Source: CAD feature listing. Evaluate the final solid. Frame: model axes, mm. Face numbers are marked on the shaded views. Coordinates: 2 decimals unless noted, no trailing zeros. Loops run counter-clockwise (first coordinate to the right, second up) from the corner with the lowest first, then second, coordinate; pieces in that order, holes last.
Item 1: Section query B-B, the plane z = 30. Return the cut outline in (x, y), then the cut area to 3 significant figures.
Item 2: Line query: probe 1 along X at (y, z) = (26.4, 10); probe 2 along Z at (x, y) = (-0.5, 30.25); probe 3 along X at (y, z) = (31, 46.5). Output: solid intervals per line, ascending.
Item 3: Pin query (flat end, axial travel): pin 1 Ø7.5 at (x, z) = (0, 50) entering from -Y; pin 2 Ø4 at (y, z) = (29.5, 15) entering from +X; pin 3 Ø7.5 at (x, z) = (0, 10) entering from +Y; pin 4 Ø1 at (y, z) = (27, 8.5) entering from -X. Return the tip coordinate at first contact, or that it passes through.
Item 4: Section query C-C, the plane y = 29. State how many separate pieces and enclosed holes the cut face has, then the cut area to 3 significant figures.
Item 5: Section query A-A, the plane x = 0. Return the cut outline in (y, z).
Item 6: Pull-direction query (X, two-part tool) for the marked faces 1, 2 and 3; classes: +X half, -X half, draft (parallel to the pull), parting line (faces both ways), or undercut.
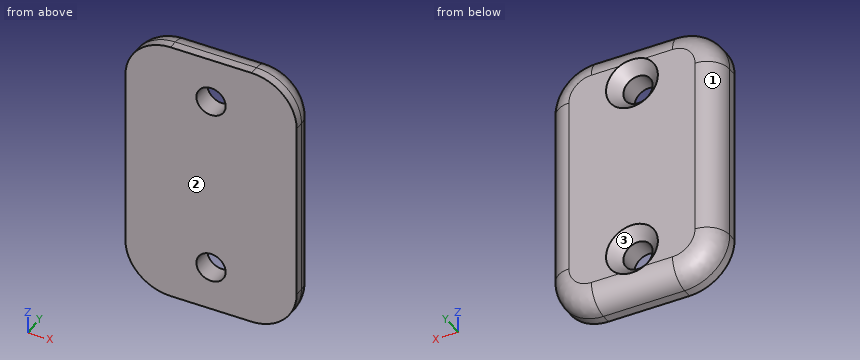
```python
from build123d import *

# Parameters (mm, degrees)
SKETCH1_W           = 43
SKETCH1_H           = 43
SKETCH1_R           = 13.75
SKETCH1_H_2         = 7
BOSS_EXTRUDE1_DEPTH = 60
SKETCH3_R           = 3.25
CUT_EXTRUDE5_DEPTH  = 85.038324591
CHAMFER2_SIZE       = 2.5
CUT_EXTRUDE6_START  = -38
CUT_EXTRUDE6_DEPTH  = 15
SKETCH9_W           = 10
SKETCH9_H           = 51.2
CUT_EXTRUDE7_DEPTH  = 75.012431469
FILLET1_R           = 5
FILLET2_R           = 10


with BuildPart() as part:
    # Sketch1 → Boss-Extrude1 (new body)
    # profile 1 of 3: a face of its own
    with BuildSketch(Plane.XY):
        with Locations((2.5, 2.5)):
            Rectangle(SKETCH1_W, SKETCH1_H)
        Circle(SKETCH1_R, mode=Mode.SUBTRACT)
    # profile 2 of 3: a face of its own
    with BuildSketch(Plane.XY):
        with Locations((2.5, 28.7)):
            Rectangle(SKETCH1_W, SKETCH1_H_2)
    # profile 3 of 3: a face of its own
    with BuildSketch(Plane.XY):
        Polygon((24, 24), (24, -19), (29, -19), (29, 32.2), (24, 32.2), (24, 25.2), align=None)
    extrude(amount=BOSS_EXTRUDE1_DEPTH)

    # Sketch3 → Cut-Extrude5 (cut, through all)
    with BuildSketch(Plane(origin=(0, 32.2, 0), x_dir=(1, 0, 0), z_dir=(0, 1, 0))):
        with Locations(Location((0, -50, 0), (0, 0, 270))):
            Circle(SKETCH3_R)
        with Locations(Location((0, -10, 0), (0, 0, 270))):
            Circle(SKETCH3_R)
    extrude(amount=-CUT_EXTRUDE5_DEPTH, mode=Mode.SUBTRACT)

    # Chamfer2
    chamfer2_edges = [part.edges().sort_by_distance(p)[0] for p in [
        (0, 32.2, 46.75),
        (0, 32.2, 6.75),
    ]]
    chamfer(chamfer2_edges, length=CHAMFER2_SIZE)

    # Sketch7 → Cut-Extrude6 (cut)
    with BuildSketch(Plane.XZ.offset(19).offset(CUT_EXTRUDE6_START)):
        Polygon((0, 43.533676985), (5.6, 46.766838493), (5.6, 53.233161507), (0, 56.466323015), (-5.6, 53.233161507), (-5.6, 46.766838493), align=None)
        Polygon((-5.6, 13.233161507), (0, 16.466323015), (5.6, 13.233161507), (5.6, 6.766838493), (0, 3.533676985), (-5.6, 6.766838493), align=None)
    extrude(amount=CUT_EXTRUDE6_DEPTH, mode=Mode.SUBTRACT)

    # Sketch9 → Cut-Extrude7 (cut, through all)
    with BuildSketch(Plane(origin=(0, 0, 0), x_dir=(-1, 0, 0), z_dir=(0, 0, -1))):
        with Locations((-24, 6.6)):
            Rectangle(SKETCH9_W, SKETCH9_H)
    extrude(amount=-CUT_EXTRUDE7_DEPTH, mode=Mode.SUBTRACT)


with BuildPart() as body_2:
    # of the pieces the cut leaves, the one that is kept (cut_extrude7_keep)
    add(part.part.solids().sort_by_distance((-19, 32.2, 0))[0])

    # Fillet1
    # the kernel refuses this fillet: 5 mm, written as the material it takes off along each edge
    with BuildSketch(Plane(origin=(-31.5, 32.2, 0), x_dir=(0, 0, 1), z_dir=(1, 0, 0)), Plane(origin=(31.5, 32.2, 60), x_dir=(0, 0, -1), z_dir=(-1, 0, 0))) as fillet1_piece_1:
        with BuildLine():
            CenterArc((FILLET1_R, FILLET1_R), FILLET1_R, 180, 90)
            Line((0, FILLET1_R), (0, 0))
            Line((0, 0), (FILLET1_R, 0))
        make_face()
    extrude(amount=63, mode=Mode.SUBTRACT)
    with BuildSketch(Plane(origin=(-19, 32.2, -12.5), x_dir=(1, 0, 0), z_dir=(0, 0, 1))) as fillet1_piece_2:
        with BuildLine():
            CenterArc((FILLET1_R, -FILLET1_R), FILLET1_R, 90, 90)
            Line((0, -FILLET1_R), (0, 0))
            Line((0, 0), (FILLET1_R, 0))
        make_face()
    extrude(amount=85, mode=Mode.SUBTRACT)
    with BuildSketch(Plane(origin=(19, 32.2, -12.5), x_dir=(-1, 0, 0), z_dir=(0, 0, 1))) as fillet1_piece_3:
        with BuildLine():
            CenterArc((FILLET1_R, FILLET1_R), FILLET1_R, 180, 90)
            Line((0, FILLET1_R), (0, 0))
            Line((0, 0), (FILLET1_R, 0))
        make_face()
    extrude(amount=85, mode=Mode.SUBTRACT)

    # Fillet2
    # the kernel refuses this fillet: 10 mm, written as the material it takes off along each edge
    with BuildSketch(Plane(origin=(-9, 32.2, 10), x_dir=(0, 0, -1), z_dir=(1, 0, 0))) as fillet2_piece_1:
        with BuildLine():
            CenterArc((5, -5), 5, 0, 90)
            Line((10, -5), (10, 0))
            Line((10, 0), (5, 0))
        make_face()
    revolve(axis=Axis((-9, 32.2, 10), (0, 1, 0)), revolution_arc=90, mode=Mode.SUBTRACT)
    with BuildSketch(Plane(origin=(9, 32.2, 10), x_dir=(1, 0, 0), z_dir=(0, 0, 1))) as fillet2_piece_2:
        with BuildLine():
            CenterArc((5, -5), 5, 0, 90)
            Line((10, -5), (10, 0))
            Line((10, 0), (5, 0))
        make_face()
    revolve(axis=Axis((9, 32.2, 10), (0, 1, 0)), revolution_arc=90, mode=Mode.SUBTRACT)
    with BuildSketch(Plane(origin=(-9, 32.2, 50), x_dir=(-1, 0, 0), z_dir=(0, 0, -1))) as fillet2_piece_3:
        with BuildLine():
            CenterArc((5, -5), 5, 0, 90)
            Line((10, -5), (10, 0))
            Line((10, 0), (5, 0))
        make_face()
    revolve(axis=Axis((-9, 32.2, 50), (0, 1, 0)), revolution_arc=90, mode=Mode.SUBTRACT)
    with BuildSketch(Plane(origin=(9, 32.2, 50), x_dir=(0, 0, 1), z_dir=(-1, 0, 0))) as fillet2_piece_4:
        with BuildLine():
            CenterArc((5, -5), 5, 0, 90)
            Line((10, -5), (10, 0))
            Line((10, 0), (5, 0))
        make_face()
    revolve(axis=Axis((9, 32.2, 50), (0, 1, 0)), revolution_arc=90, mode=Mode.SUBTRACT)
    with BuildSketch(Plane(origin=(19, 32.2, 0), x_dir=(0, 0, 1), z_dir=(0, -1, 0)), Plane(origin=(-19, 32.2, 60), x_dir=(0, 0, -1), z_dir=(0, -1, 0))) as fillet2_piece_5:
        with BuildLine():
            CenterArc((FILLET2_R, FILLET2_R), FILLET2_R, 180, 90)
            Line((0, FILLET2_R), (0, 0))
            Line((0, 0), (FILLET2_R, 0))
        make_face()
    extrude(amount=32, mode=Mode.SUBTRACT)
    with BuildSketch(Plane(origin=(19, 0.2, 60), x_dir=(-1, 0, 0), z_dir=(0, 1, 0)), Plane(origin=(-19, 32.2, 0), x_dir=(0, 0, 1), z_dir=(0, -1, 0))) as fillet2_piece_6:
        with BuildLine():
            CenterArc((FILLET2_R, -FILLET2_R), FILLET2_R, 90, 90)
            Line((0, -FILLET2_R), (0, 0))
            Line((0, 0), (FILLET2_R, 0))
        make_face()
    extrude(amount=32, mode=Mode.SUBTRACT)


solid = body_2.part
```
Verdict:
1. outline: (-19, 25.2) - (19, 25.2) - (19, 27.2) arc R5 ccw to (14, 32.2) - (-14, 32.2) arc R5 ccw to (-19, 27.2) - close
1. area: 255 mm2
2. probe 1: x = -19 to -3.25, 3.25 to 19
2. probe 2: z = 1.04 to 6.23, 13.77 to 46.23, 53.77 to 58.96
2. probe 3: x = -17.25 to -2.91, 2.91 to 17.25
3. pin 1: stops at y = 25.2
3. pin 2: stops at x = 18.99
3. pin 3: stops at y = 30.2
3. pin 4: stops at x = -18.95
4. separate pieces: 1
4. enclosed holes: 2
4. area: 2,070 mm2
5. outline: (25.2, 0) - (27.2, 0) arc R5 ccw to (32.15, 4.3) - (29.7, 6.75) - (25.2, 6.75) - close; (25.2, 13.25) - (29.7, 13.25) - (32.2, 15.75) - (32.2, 44.25) - (29.7, 46.75) - (25.2, 46.75) - close; (25.2, 53.25) - (29.7, 53.25) - (32.15, 55.7) arc R5 ccw to (27.2, 60) - (25.2, 60) - close
6. face 1: -X half
6. face 2: draft
6. face 3: undercut
